```python
from build123d import *

# Parameters (mm, degrees)
SKETCH1_R           = 4
BOSS_EXTRUDE1_DEPTH = 16
CUT_EXTRUDE1_DEPTH  = 55.598534779


with BuildPart() as part:
    # Sketch1 → Boss-Extrude1 (new body)
    with BuildSketch(Plane.XY):
        with BuildLine():
            Line((8, 0), (8, -15))
            ThreePointArc((8, -15), (5.656854249, -20.656854249), (0, -23))
            Line((0, -23), (-42, -23))
            Line((-42, -23), (-42, 8))
            Line((-42, 8), (0, 8))
            ThreePointArc((0, 8), (5.656854249, 5.656854249), (8, 0))
        make_face()
        Circle(SKETCH1_R, mode=Mode.SUBTRACT)
        with Locations((0, -15)):
            Circle(SKETCH1_R, mode=Mode.SUBTRACT)
    extrude(amount=-BOSS_EXTRUDE1_DEPTH)

    # Sketch2 → Cut-Extrude1 (cut, through all)
    with BuildSketch(Plane(origin=(0, 8, 0), x_dir=(1, 0, 0), z_dir=(0, 1, 0))):
        with BuildLine():
            Line((-34, 12), (-12, 12))
            ThreePointArc((-12, 12), (-8, 8), (-12, 4))
            Line((-12, 4), (-34, 4))
            ThreePointArc((-34, 4), (-38, 8), (-34, 12))
        make_face()
    extrude(amount=-CUT_EXTRUDE1_DEPTH, mode=Mode.SUBTRACT)


solid = part.part
```
Could you check a few things on this model? Use its own coordinates, in mm. A direction names the side the tool comes from. Coordinates: 2 decimals unless noted, no trailing zeros. Write each loop counter-clockwise with the first axis right and the second up, starting at its lowest first coordinate (ties: lowest second). Pieces come first, ordered by that corner, then holes. Notation, with made-up numbers: (55, 50) -> (88, 50) arc R20 ccw to (88, 61) -> close; hole circle Ø11 at (32.5, 78). An arc over 180 degrees is marked (long way). One line per question, with ' | ' between items. Start each with the question number.
1. If we section it at B-B (y = 3.5): Please give me the cut outline in (x, z).
2. Will these pins go through, and if not, where does the flat tip stop? P1, Ø3, axis at x = -35, y = -9, coming from the +Z side; P2, Ø5, axis at x = 0, y = 0, coming from the +Z side.
3. Please list where these lines run through material, in increasing order: line 1 along Y through (x, z) = (0, -4.25); line 2 along Z through (x, y) = (-29.5, -7.5); line 3 along X through (y, z) = (-3.5, -11.25).
4. For faces 1 (the face through (-38, -7, -8)), 2 (the face through (-17, -7, 0)), which set-ups out of +Z, -Z, +X, -X, +Y, -Y let a thin tool reach every point of the face, with its end or its side?
5. Thinking about a two-plate mould opening in Y: for faces 3 (the face through (-42, -8, -8)), 4 (the face through (-0.521, -11.034, -7.888)), 5 (the face through (-21, -23, -13)), 6 (the face through (5.594, 5.719, -7.888)), which applies, pulls with the +Y half, pulls with the -Y half, needs draft (parallel to the pull), parting line crosses it, or undercut?
6. If we section it at C-C (x = -34.5): Please give me the cut outline in (y, z).
7. If we section it at A-A (z = -8): Please give me the cut outline in (x, y), and give its area (3 significant figures).
8. If we section it at D-D (z = -1.75): Please give me the cut outline in (x, y).
Return value:
1) outline: (-42, -16) -> (-1.94, -16) -> (-1.94, 0) -> (-42, 0) -> close; (1.94, -16) -> (7.19, -16) -> (7.19, 0) -> (1.94, 0) -> close; hole (-34, -12) -> (-12, -12) arc R4 ccw to (-12, -4) -> (-34, -4) arc R4 ccw to start
2) P1: stops at z = 0 | P2: passes through
3) line 1: y = -23 to -19, -11 to -4, 4 to 8 | line 2: z = -16 to -12, -4 to 0 | line 3: x = -42 to -36.33, -9.67 to -1.94, 1.94 to 8
4) face 1: +Y, -Y | face 2: +Z, +X, -X, +Y, -Y
5) face 3: needs draft | face 4: undercut | face 5: pulls with the -Y half | face 6: pulls with the +Y half
6) outline: (-23, -16) -> (8, -16) -> (8, -11.97) -> (-23, -11.97) -> close; (-23, -4.03) -> (8, -4.03) -> (8, 0) -> (-23, 0) -> close
7) outline: (-42, -23) -> (-38, -23) -> (-38, 8) -> (-42, 8) -> close; (-8, -23) -> (0, -23) arc R8 ccw to (8, -15) -> (8, 0) arc R8 ccw to (0, 8) -> (-8, 8) -> close; hole circle Ø8 at (0, -15); hole circle Ø8 at (0, 0) | area: 492 mm²
8) outline: (-42, -23) -> (0, -23) arc R8 ccw to (8, -15) -> (8, 0) arc R8 ccw to (0, 8) -> (-42, 8) -> close; hole circle Ø8 at (0, -15); hole circle Ø8 at (0, 0)
